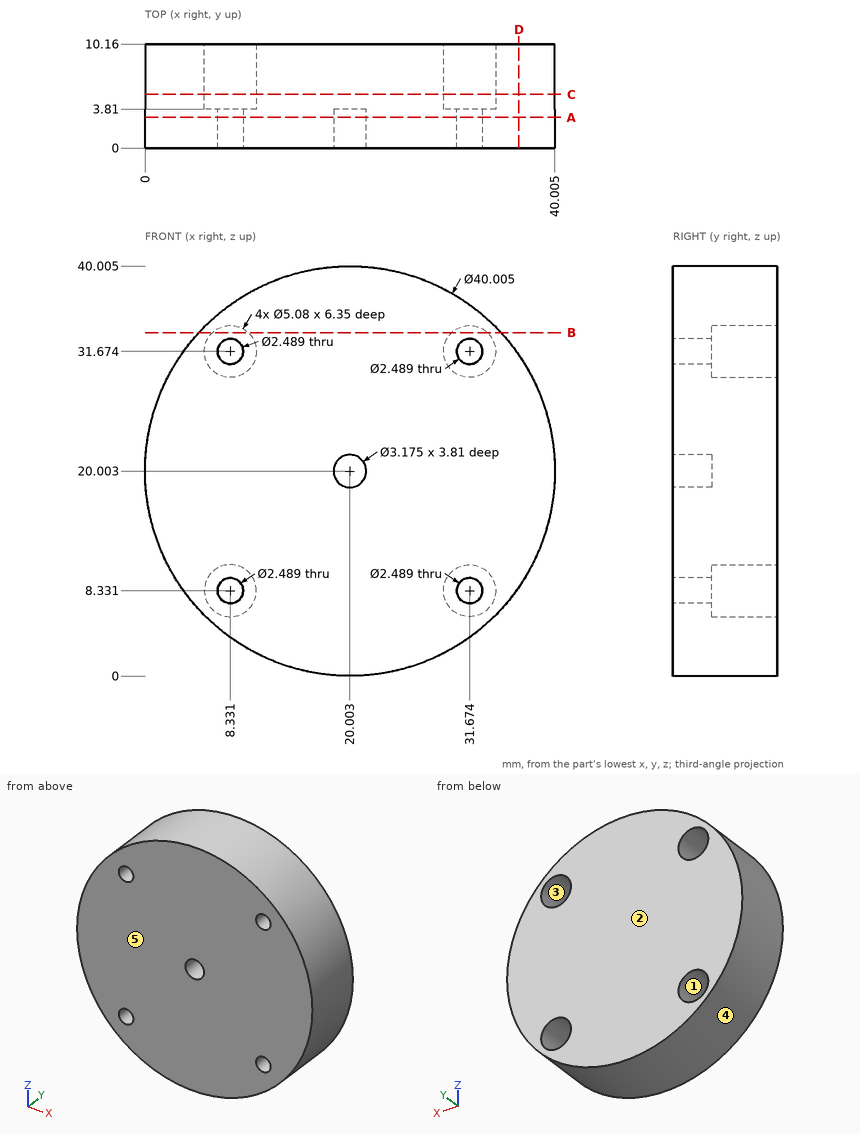
Job drawing, mm, ordinate dimensions from the low corner. One solid piece. A direction names the side the tool comes from. Give positions to 0.01 mm unless a question says otherwise; leave off trailing zeros. Write each loop counter-clockwise with the first axis right and the second up, starting at its lowest first coordinate (ties: lowest second). Pieces come first, ordered by that corner, then holes. Notation, with made-up numbers: (80, -18.75) - (125, -18.75) arc R27 ccw to (125, 15.25) - close; hole circle Ø1 at (67, 33). An arc over 180 degrees is marked (long way). Use one line per item in the form item = value. Start each with the question number.
1. Probe line 1 (Z direction, x = 9, y = 5.5) (1 decimal); line 2 (Z direction, x = 7, y = 7.25) (1 decimal); line 3 (X direction, y = 6, z = 10) (1 decimal). List the from-to ranges inside material, lowest first. Write a range as [from, to].
2. Drop flat-ended pins along their axis: pin 1 Ø12 at (x, z) = (13.5, 22.5) entering from -Y; pin 2 Ø2.5 at (x, z) = (31.5, 32.5) entering from +Y; pin 3 Ø3 at (x, y) = (17.5, 8.5) entering from -Z (1 decimal); pin 4 Ø1 at (x, y) = (30, 8) entering from -Z. Give the stop position or say it passes through.
3. Band-saw the part on D-D on x = 36.5. Write the cut outline in (y, z).
4. 3-axis set-ups, long thin cutter, end or side, ignore diameter. For the marked faces 1 and 2: which of +Z, -Z, +X, -X, +Y, -Y reach the whole face in a straight line?
5. Two-plate mould, pull along Z, no slides. Class the marked faces 3, 4 and 5: released by +Z, released by -Z, zero draft, split by the parting line, or undercut.
6. Band-saw the part on A-A on y = 3. Write the cut outline in (x, z) (1 decimal), plus the area to 3 significant figures.
7. Band-saw the part on B-B on z = 33.5. Write the cut outline in (x, y) (1 decimal).
8. Band-saw the part on C-C on y = 5.25. Write the cut outline in (x, z) (1 decimal), plus the area to 3 significant figures.
Conclusion:
q1.line_1 = [3.3, 5.9], [10.8, 29.2], [34.1, 36.7]
q1.line_2 = [4.8, 6.2], [10.5, 29.5], [33.8, 35.2]
q1.line_3 = [2.7, 6.4], [10.2, 29.8], [33.6, 37.3]
q2.pin_1 = 0
q2.pin_2 = 3.81
q2.pin_3 = 0
q2.pin_4 = 2.4
q3.outline = (0, 8.69) - (10.16, 8.69) - (10.16, 31.31) - (0, 31.31) - close
q4.face_1 = +Y
q4.face_2 = +Z, -Z, +X, -X, +Y
q5.face_3 = undercut
q5.face_4 = split by the parting line
q5.face_5 = zero draft
q6.outline = circle Ø40 at (20, 20); hole circle Ø2.5 at (8.3, 8.3); hole circle Ø2.5 at (8.3, 31.7); hole circle Ø3.2 at (20, 20); hole circle Ø2.5 at (31.7, 8.3); hole circle Ø2.5 at (31.7, 31.7)
q6.area = 1,230 mm²
q7.outline = (5.2, 0) - (34.8, 0) - (34.8, 10.2) - (33.4, 10.2) - (33.4, 3.8) - (29.9, 3.8) - (29.9, 10.2) - (10.1, 10.2) - (10.1, 3.8) - (6.6, 3.8) - (6.6, 10.2) - (5.2, 10.2) - close
q8.outline = circle Ø40 at (20, 20); hole circle Ø5.1 at (8.3, 8.3); hole circle Ø5.1 at (8.3, 31.7); hole circle Ø5.1 at (31.7, 8.3); hole circle Ø5.1 at (31.7, 31.7)
q8.area = 1,180 mm²
